Geometry check sheet. Reference: the model listing, model coordinates, mm. Face numbers are marked on the shaded views. A direction names the side the tool comes from. Round coordinates to 2 decimals unless told otherwise and drop trailing zeros. Write each loop counter-clockwise with the first axis right and the second up, starting at its lowest first coordinate (ties: lowest second). Pieces come first, ordered by that corner, then holes. Notation, with made-up numbers: (84, -28.5) - (104, -28.5) arc R4 ccw to (104, -21.5) - close; hole circle Ø3 at (45, 51). An arc over 180 degrees is marked (long way). Return JSON: item names as keys, results as strings. Group by question number.
from build123d import *

# Parameters (mm, degrees)
BOSS_EXTRUDE1_DEPTH = 6.35


with BuildPart() as part:
    # Sketch1 → Boss-Extrude1 (new body)
    with BuildSketch(Plane(origin=(0, 0, 0), x_dir=(1, 0, 0), z_dir=(0, 1, 0))):
        with BuildLine():
            Line((26.67, 7.62), (26.67, 15.24))
            ThreePointArc((26.67, 15.24), (25.182102448, 18.832102448), (21.59, 20.32))
            Line((21.59, 20.32), (-21.59, 20.32))
            ThreePointArc((-21.59, 20.32), (-25.182102448, 18.832102448), (-26.67, 15.24))
            Line((-26.67, 15.24), (-26.67, -40.64))
            ThreePointArc((-26.67, -40.64), (-25.182102448, -44.232102448), (-21.59, -45.72))
            Line((-21.59, -45.72), (5.08, -45.72))
            ThreePointArc((5.08, -45.72), (7.780244368, -44.942915332), (9.654379091, -42.849401713))
            Line((9.654379091, -42.849401713), (26.67, -7.62))
            Line((26.67, -7.62), (26.67, 0))
            Line((26.67, 0), (0, 0))
            Line((0, 0), (0, 7.62))
            Line((0, 7.62), (26.67, 7.62))
        make_face()
    extrude(amount=BOSS_EXTRUDE1_DEPTH)


solid = part.part
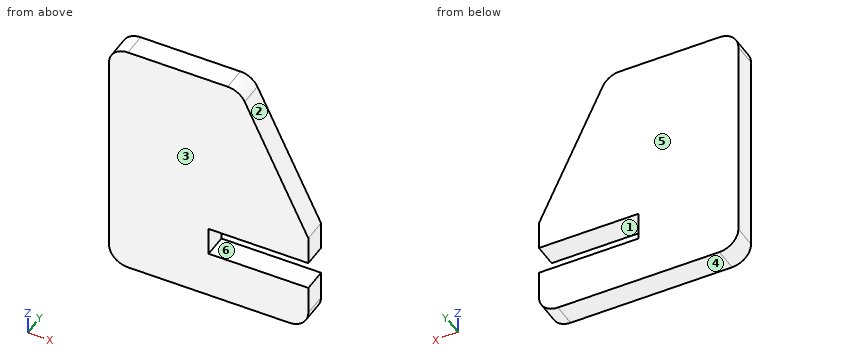
1. Tool access check on the marked faces 5 and 6. Record the directions out of +Z, -Z, +X, -X, +Y, -Y that give a thin tool (end or side, any length) a straight path to the whole face; none if there is none.
2. Mould release check, pull along Z, two halves, no side actions. Record for the marked faces 1, 2, 3 and 4: pulls with the +Z half, pulls with the -Z half, needs draft (parallel to the pull), parting line crosses it, or undercut.
3. Section check A-A (x = 11.5). Enter the section's corners in (y, z).
4. Material ranges on line 1 along X through (y, z) = (2.25, -5.5); line 2 along Z through (x, y) = (23, 1); line 3 along Z through (x, y) = (8, 2.5), recorded low to high.
5. Section check D-D (z = 17.5). Enter the section's corners in (x, y), and give its area (3 significant figures).
6. Section check B-B (y = 2.25). Enter the section's corners in (x, z), and give its area (3 significant figures).
7. Section check C-C (z = 37.5). Enter the section's corners in (x, y).
8. Depth check by flat-ended pin: pin 1 Ø1.5 at (y, z) = (2.5, 22) entering from +X; pin 2 Ø2 at (y, z) = (5.5, 12.5) entering from +X; pin 3 Ø2 at (x, z) = (-14, -5) entering from -Y. Enter the tip coordinate at first touch or a pass-through.
Result sheet:
{
 "1": {"face 5": "+Z, -Z, +X, -X, +Y", "face 6": "+X, +Y, -Y"},
 "2": {"face 1": "undercut", "face 2": "pulls with the +Z half", "face 3": "needs draft", "face 4": "pulls with the -Z half"},
 "3": {"outline": "(0, -20.32) - (6.35, -20.32) - (6.35, -7.62) - (0, -7.62) - close; (0, 0) - (6.35, 0) - (6.35, 39.03) - (0, 39.03) - close"},
 "4": {"line 1": "x = -26.67 to 0", "line 2": "z = -20.12 to -7.62, 0 to 15.22", "line 3": "z = -20.32 to -7.62, 0 to 44.8"},
 "5": {"outline": "(-26.67, 0) - (21.9, 0) - (21.9, 6.35) - (-26.67, 6.35) - close", "area": "308 mm²"},
 "6": {"outline": "(-26.67, -15.24) arc R5.08 ccw to (-21.59, -20.32) - (21.59, -20.32) arc R5.08 ccw to (26.67, -15.24) - (26.67, -7.62) - (0, -7.62) - (0, 0) - (26.67, 0) - (26.67, 7.62) - (9.65, 42.85) arc R5.08 ccw to (5.08, 45.72) - (-21.59, 45.72) arc R5.08 ccw to (-26.67, 40.64) - close", "area": "2,950 mm²"},
 "7": {"outline": "(-26.67, 0) - (12.24, 0) - (12.24, 6.35) - (-26.67, 6.35) - close"},
 "8": {"pin 1": "stops at x = 20.09", "pin 2": "stops at x = 24.8", "pin 3": "stops at y = 0"}
}
